Can you work these out from the model? Positions are in its coordinate system, mm. Face numbers are marked on the shaded views. A direction names the side the tool comes from. Give positions to 0.01 mm unless a question says otherwise; leave off trailing zeros. Write each loop counter-clockwise with the first axis right and the second up, starting at its lowest first coordinate (ties: lowest second). Pieces come first, ordered by that corner, then holes. Notation, with made-up numbers: (-28.5, 5) -> (-16.5, 5) arc R15 ccw to (-16.5, 13) -> close; hole circle Ø5 at (-16.5, 72.5). An arc over 180 degrees is marked (long way). One line per item, written item: value.
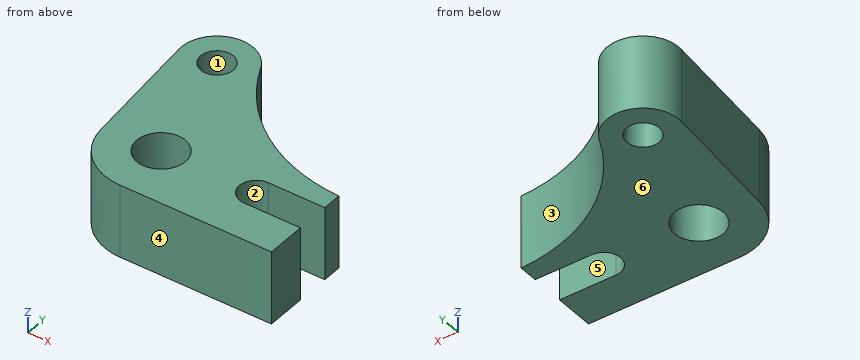
from build123d import *

# Parameters (mm, degrees)
ESQUISSE1_R        = 9.5
ESQUISSE1_R_2      = 6.35
BOSS_EXTRU_3_DEPTH = 28.5


with BuildPart() as part:
    # Esquisse1 → Boss.-Extru.3 (new body)
    with BuildSketch(Plane.XY):
        with BuildLine():
            Line((-32.183370977, -41.533470352), (26.816629023, -41.533470352))
            Line((26.816629023, -41.533470352), (26.816629023, -26.033470352))
            Line((26.816629023, -26.033470352), (4.816629023, -26.033470352))
            ThreePointArc((4.816629023, -26.033470352), (-1.683370977, -19.533470352), (4.816629023, -13.033470352))
            Line((4.816629023, -13.033470352), (26.816629023, -13.033470352))
            Line((26.816629023, -13.033470352), (26.816629023, -5.533470352))
            ThreePointArc((26.816629023, -5.533470352), (-8.245750613, 5.622429434), (-32.129953671, 33.611166634))
            ThreePointArc((-32.129953671, 33.611166634), (-48.50573191, 41.315354446), (-58.798603767, 26.429877911))
            Line((-58.798603767, 26.429877911), (-54.078241746, -21.681640278))
            ThreePointArc((-54.078241746, -21.681640278), (-46.960722933, -35.831625744), (-32.183370977, -41.533470352))
        make_face()
        with Locations(Location((-32.183370977, -19.533470352, 0), (0, 0, 180))):
            Circle(ESQUISSE1_R, mode=Mode.SUBTRACT)
        with Locations(Location((-44.865504187, 27.796895136, 0), (0, 0, 180))):
            Circle(ESQUISSE1_R_2, mode=Mode.SUBTRACT)
    extrude(amount=BOSS_EXTRU_3_DEPTH)


solid = part.part
1) If we section it at A-A (x = -47.5): Write out the boundary of the cut face in (y, z), and give its area (3 significant figures).
Answer list:
outline: (-35.33, 0) -> (22.02, 0) -> (22.02, 28.5) -> (-35.33, 28.5) -> close; (33.57, 0) -> (41.55, 0) -> (41.55, 28.5) -> (33.57, 28.5) -> close
area: 1,860 mm^2
2) I need wall thicknesses on L1, parallel to Y at x = -39, z = 16.75; L2, parallel to Y at x = -29, z = 25.5; L3, parallel to Y at x = 0, z = 11. Which ranges of each line are inside material? Lowest first, please.
Answer list:
L1: y = -40.45 to -26.15, -12.92 to 25.36, 30.23 to 40.51
L2: y = -41.53 to -28.48, -10.58 to 27.58
L3: y = -41.53 to -23.9, -15.17 to 0.95
3) If we section it at B-B (z = 23.25): Write out the boundary of the cut face in (x, y), and give its area (3 significant figures).
Answer list:
outline: (-58.8, 26.43) -> (-54.08, -21.68) arc R22 ccw to (-32.18, -41.53) -> (26.82, -41.53) -> (26.82, -26.03) -> (4.82, -26.03) arc R6.5 cw to (4.82, -13.03) -> (26.82, -13.03) -> (26.82, -5.53) arc R67 cw to (-32.13, 33.61) arc R14 ccw to start; hole circle Ø12.7 at (-44.87, 27.8); hole circle Ø19 at (-32.18, -19.53)
area: 3,870 mm^2
4) Will these pins go through, and if not, where does the flat tip stop? pin 1 (8 mm diameter, centred on x = -47.5, z = 8, fed in from -Y); pin 2 (1.5 mm diameter, centred on x = -32.5, z = 19, fed in from +Y); pin 3 (6 mm diameter, centred on y = 24.5, z = 19, fed in from +X).
Answer list:
pin 1: stops at y = -38.4
pin 2: stops at y = 35.61
pin 3: stops at x = -24.98
5) We'd pull the mould along Y, two halves only. Please class the marked faces 1, 2, 3 and 4: released by +Y, released by -Y, zero draft, split by the parting line, or undercut.
Answer list:
face 1: undercut
face 2: undercut
face 3: released by +Y
face 4: released by -Y
6) If we section it at D-D (y = 10): Write out the boundary of the cut face in (x, z).
Answer list:
outline: (-57.19, 0) -> (-14.11, 0) -> (-14.11, 28.5) -> (-57.19, 28.5) -> close
7) If we section it at C-C (x = -29): Write out the boundary of the cut face in (y, z), and give its area (3 significant figures).
Answer list:
outline: (-41.53, 0) -> (-28.48, 0) -> (-28.48, 28.5) -> (-41.53, 28.5) -> close; (-10.58, 0) -> (27.58, 0) -> (27.58, 28.5) -> (-10.58, 28.5) -> close
area: 1,460 mm^2
8) For the marked faces 5 and 6, which set-ups out of +Z, -Z, +X, -X, +Y, -Y let a thin tool reach every point of the face, with its end or its side?
Answer list:
face 5: +Z, -Z, +X
face 6: -Z, +X, -X, +Y, -Y
